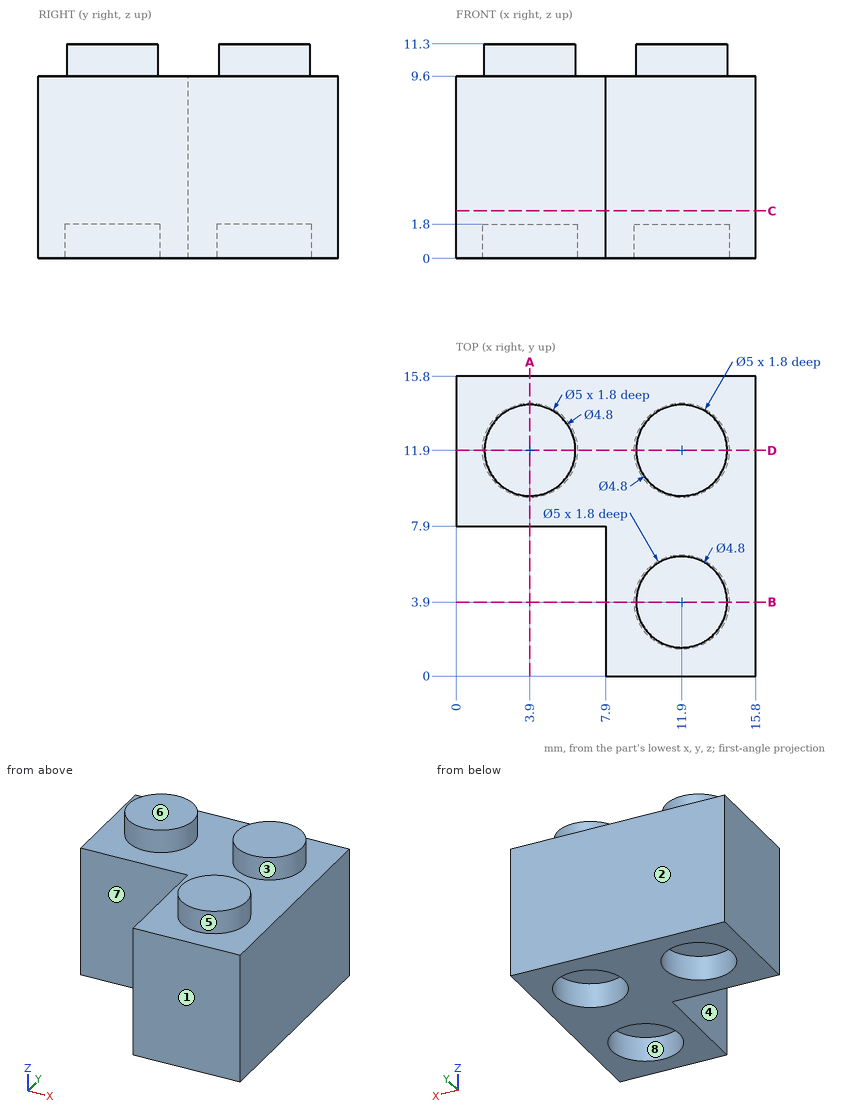
Here's the drawing with two shaded views (mm, measured from the low corner). I have some questions. A direction names the side the tool comes from. Give positions to 0.01 mm unless a question says otherwise; leave off trailing zeros. Loops run counter-clockwise (first coordinate to the right, second up) from the corner with the lowest first, then second, coordinate; pieces in that order, holes last. Notation, with made-up numbers: M -36.75,5 L -7.75,5 A28 cw -7.75,34 Z; hole C -11.75,7.25 d5. An arc over 180 degrees is marked long. One line per item, written item: value. Start each with the question number.
1) If I drill on line 1 (Y direction, x = 11.9, z = 0.75); line 2 (Z direction, x = 11.25, y = 5); line 3 (Y direction, x = 3.9, z = 1.1), over which ranges is the centre line in solid material (lowest first)? Write a range as [from, to].
2) If we section it at C-C, the plane z = 2.5: Write out the boundary of the cut face in (x, y), and give its area (3 significant figures).
3) Thinking about a two-plate mould opening in Y: for the marked faces 1, 2, 3 and 4, which applies, +Y half, -Y half, draft (parallel to the pull), parting line (faces both ways), or undercut?
4) If we section it at A-A, the plane x = 3.9: Write out the boundary of the cut face in (y, z), and give its area (3 significant figures).
5) I'm going to push flat-ended pins straight in: pin 1 (1.5 mm diameter, centred on x = 2.5, y = 10.5, fed in from -Z); pin 2 (6.5 mm diameter, centred on x = 2.5, z = 5.5, fed in from -Y); pin 3 (4 mm diameter, centred on x = 3.9, y = 11.9, fed in from -Z); pin 4 (3 mm diameter, centred on y = 3, z = 3, fed in from -X). Where does each tip first touch, or does it pass through?
6) On a 3-axis mill with a long thin cutter (end or side, diameter ignored), from which of +Z, -Z, +X, -X, +Y, -Y can I reach the whole of each face in a straight line? I mean the marked faces 5, 6, 7 and 8. Say none if no direction works.
7) If we section it at D-D, the plane y = 11.9: Write out the boundary of the cut face in (x, z).
Completed:
1. line 1: y = [0, 1.4], [6.4, 9.4], [14.4, 15.8]
1. line 2: z = [1.8, 11.3]
1. line 3: y = [7.9, 9.4], [14.4, 15.8]
2. outline: M 0,7.9 L 7.9,7.9 L 7.9,0 L 15.8,0 L 15.8,15.8 L 0,15.8 Z
2. area: 187 mm^2
3. face 1: -Y half
3. face 2: +Y half
3. face 3: undercut
3. face 4: draft
4. outline: M 7.9,0 L 9.4,0 L 9.4,1.8 L 14.4,1.8 L 14.4,0 L 15.8,0 L 15.8,9.6 L 14.3,9.6 L 14.3,11.3 L 9.5,11.3 L 9.5,9.6 L 7.9,9.6 Z
4. area: 75.0 mm^2
5. pin 1: stops at z = 0
5. pin 2: stops at y = 7.9
5. pin 3: stops at z = 1.8
5. pin 4: stops at x = 7.9
6. face 5: +Z
6. face 6: +Z, +X, -X, +Y, -Y
6. face 7: +Z, -Z, -X, -Y
6. face 8: -Z
7. outline: M 0,0 L 1.4,0 L 1.4,1.8 L 6.4,1.8 L 6.4,0 L 9.4,0 L 9.4,1.8 L 14.4,1.8 L 14.4,0 L 15.8,0 L 15.8,9.6 L 14.3,9.6 L 14.3,11.3 L 9.5,11.3 L 9.5,9.6 L 6.3,9.6 L 6.3,11.3 L 1.5,11.3 L 1.5,9.6 L 0,9.6 Z
